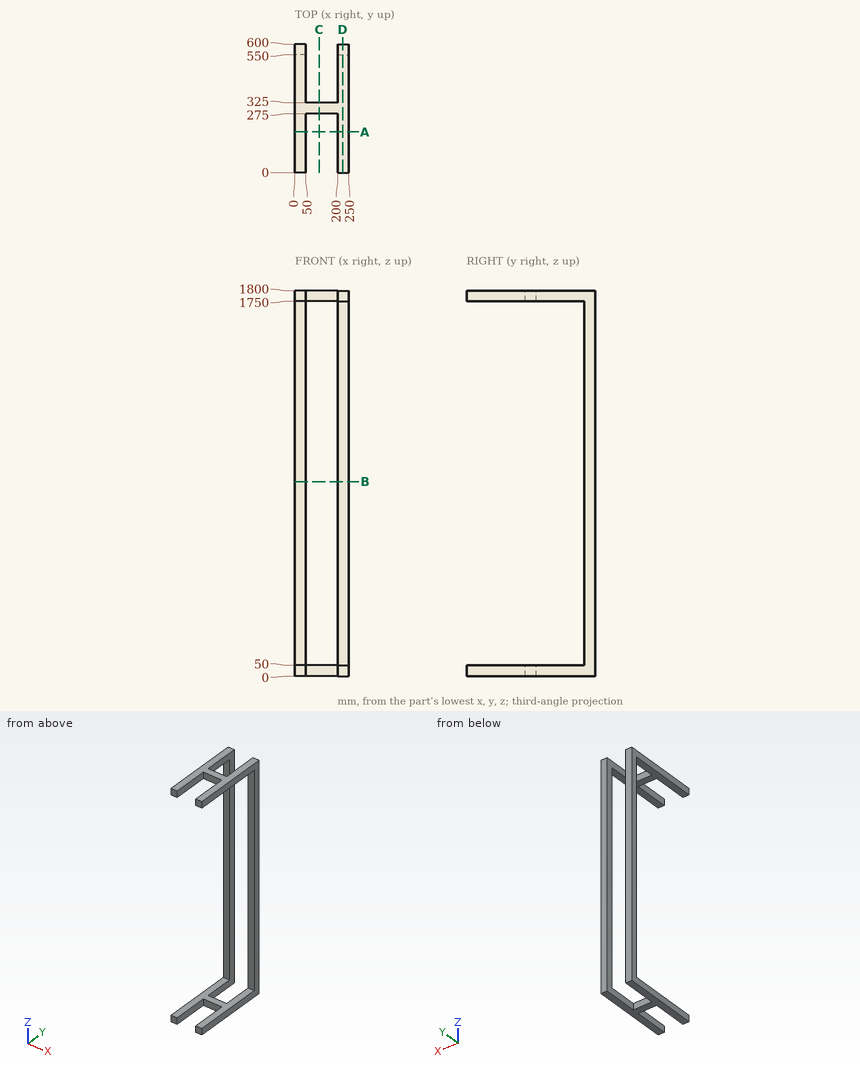
Here's the drawing with two shaded views (mm, measured from the low corner). I have some questions. Round coordinates to 2 decimals unless told otherwise and drop trailing zeros. Loops run counter-clockwise (first coordinate to the right, second up) from the corner with the lowest first, then second, coordinate; pieces in that order, holes last. Notation, with made-up numbers: M 85.5,85 L 110.5,85 A21 ccw 110.5,111 Z; hole C -5,72 d5. An arc over 180 degrees is marked long. Answer as a JSON object with one key per item and string values. Group by question number.
Q1. Imagine slicing it at C-C, the plane x = 112.5. Please give me the cut outline in (y, z), then the cut area to 3 significant figures.
Q2. Imagine slicing it at A-A, the plane y = 190. Please give me the cut outline in (x, z), then the cut area to 3 significant figures.
Q3. Please list where these lines run through material, in increasing order: L1, parallel to X at y = 557.5, z = 206; L2, parallel to Z at x = 214.5, y = 26.5; L3, parallel to Y at x = 42, z = 319.
Q4. Will these pins go through, and if not, where does the flat tip stop? pin 1 (25 mm diameter, centred on x = 216, z = 1178, fed in from -Y); pin 2 (15 mm diameter, centred on x = 122.5, z = 1769.5, fed in from -Y).
Q5. Imagine slicing it at B-B, the plane z = 907.5. Please give me the cut outline in (x, y), then the cut area to 3 significant figures.
Q6. Imagine slicing it at D-D, the plane x = 222.5. Please give me the cut outline in (y, z), then the cut area to 3 significant figures.
Findings:
{
 "1": {"outline": "M 275,0 L 325,0 L 325,50 L 275,50 Z; M 275,1750 L 325,1750 L 325,1800 L 275,1800 Z", "area": "5,000 mm2"},
 "2": {"outline": "M 0,0 L 50,0 L 50,50 L 0,50 Z; M 0,1750 L 50,1750 L 50,1800 L 0,1800 Z; M 200,0 L 250,0 L 250,50 L 200,50 Z; M 200,1750 L 250,1750 L 250,1800 L 200,1800 Z", "area": "10,000 mm2"},
 "3": {"L1": "x = 0 to 50, 200 to 250", "L2": "z = 0 to 50, 1750 to 1800", "L3": "y = 550 to 600"},
 "4": {"pin 1": "stops at y = 550", "pin 2": "stops at y = 275"},
 "5": {"outline": "M 0,550 L 50,550 L 50,600 L 0,600 Z; M 200,550 L 250,550 L 250,600 L 200,600 Z", "area": "5,000 mm2"},
 "6": {"outline": "M 0,0 L 600,0 L 600,1800 L 0,1800 L 0,1750 L 550,1750 L 550,50 L 0,50 Z", "area": "145,000 mm2"}
}
